from build123d import *

# Parameters (mm, degrees)
IZIM1_W                     = 15
IZIM1_H                     = 153
Y_KSEKLIK_EKSTR_ZYON1_DEPTH = 100
IZIM2_R                     = 5
KES_EKSTR_ZYON2_DEPTH       = 16
IZIM3_R                     = 16
KES_EKSTR_ZYON3_DEPTH       = 16


with BuildPart() as part:
    # Çizim1 → Yükseklik-Ekstrüzyon1 (new body)
    with BuildSketch(Plane.XY):
        Rectangle(IZIM1_W, IZIM1_H)
    extrude(amount=Y_KSEKLIK_EKSTR_ZYON1_DEPTH)

    # Çizim2 → Kes-Ekstrüzyon2 (cut, through all)
    with BuildSketch(Plane(origin=(7.5, 0, 0), x_dir=(0, 0, -1), z_dir=(1, 0, 0))):
        with Locations((-75, -69)):
            Circle(IZIM2_R)
        with Locations((-25, -69)):
            Circle(IZIM2_R)
    extrude(amount=-KES_EKSTR_ZYON2_DEPTH, mode=Mode.SUBTRACT)

    # Çizim3 → Kes-Ekstrüzyon3 (cut, through all)
    with BuildSketch(Plane(origin=(7.5, 0, 0), x_dir=(0, 0, -1), z_dir=(1, 0, 0))):
        with Locations((-50, -21.5)):
            Circle(IZIM3_R)
        with BuildLine():
            Line((-58.38409441, 35.653702621), (-41.38409441, 35.653702621))
            ThreePointArc((-41.38409441, 35.653702621), (-37.848560504, 37.118168715), (-36.38409441, 40.653702621))
            Line((-36.38409441, 40.653702621), (-36.38409441, 57.653702621))
            ThreePointArc((-36.38409441, 57.653702621), (-37.848560504, 61.189236527), (-41.38409441, 62.653702621))
            Line((-41.38409441, 62.653702621), (-58.38409441, 62.653702621))
            ThreePointArc((-58.38409441, 62.653702621), (-61.919628316, 61.189236527), (-63.38409441, 57.653702621))
            Line((-63.38409441, 57.653702621), (-63.38409441, 40.653702621))
            ThreePointArc((-63.38409441, 40.653702621), (-61.919628316, 37.118168715), (-58.38409441, 35.653702621))
        make_face()
    extrude(amount=-KES_EKSTR_ZYON3_DEPTH, mode=Mode.SUBTRACT)


solid = part.part
Could you check a few things on this model? Use its own coordinates, in mm. A direction names the side the tool comes from. Give positions to 0.01 mm unless a question says otherwise; leave off trailing zeros. Loops run counter-clockwise (first coordinate to the right, second up) from the corner with the lowest first, then second, coordinate; pieces in that order, holes last. Notation, with made-up numbers: M -34.75,88.25 L 18.25,88.25 A22 cw 18.25,108.25 Z; hole C 53.5,19.25 d1. An arc over 180 degrees is marked long. Answer as a JSON object with one key per item and string values.
Q1. Suppose I cut it at A-A, the plane z = 50. List the corners of the cut face in (x, y) for me.
Values found:
{"outline": "M -7.5,-76.5 L 7.5,-76.5 L 7.5,-37.5 L -7.5,-37.5 Z; M -7.5,-5.5 L 7.5,-5.5 L 7.5,35.65 L -7.5,35.65 Z; M -7.5,62.65 L 7.5,62.65 L 7.5,76.5 L -7.5,76.5 Z"}
Q2. For faces 4 (the flat face through (-7.5, -1, 49)), 5 (the cylindrical face through (0.11, 37.08, 37.89)), which set-ups out of +Z, -Z, +X, -X, +Y, -Y let a thin tool reach every point of the face, with its end or its side?
Values found:
{"face 4": "+Z, -Z, -X, +Y, -Y", "face 5": "+X, -X"}
Q3. For P1, Ø4, axis at x = -5.5, y = 33, coming from the -Z side, with a flat end and sliding along its axis, tell me the tip position at first contact or that it passes through.
Values found:
{"P1": "stops at z = 0"}
Q4. If we mould it in two halves opening along Z, with no side actions, what happens to faces 1 (the flat face through (0, 49, 36.384)), 2 (the flat face through (0, 1, 0)), 3 (the flat face through (0, 76.5, 49))? For each: pulls with the +Z half, pulls with the -Z half, needs draft (parallel to the pull), parting line crosses it, or undercut.
Values found:
{"face 1": "undercut", "face 2": "pulls with the -Z half", "face 3": "needs draft"}
Q5. Suppose I cut it at D-D, the plane x = -5.25. List the corners of the cut face in (y, z) for me.
Values found:
{"outline": "M -76.5,0 L 76.5,0 L 76.5,100 L -76.5,100 Z; hole C -69,25 d10; hole C -69,75 d10; hole C -21.5,50 d32; hole M 35.65,41.38 A5 ccw 40.65,36.38 L 57.65,36.38 A5 ccw 62.65,41.38 L 62.65,58.38 A5 ccw 57.65,63.38 L 40.65,63.38 A5 ccw 35.65,58.38 Z"}
Q6. If I drill on probe 1 along Y at (x, z) = (3.25, 50); probe 2 along Y at (x, z) = (-1, 41.5); probe 3 along Y at (x, z) = (3.25, 25), over which ranges is the centre line in solid material (lowest first)? Write a range as [from, to].
Values found:
{"probe 1": "y = [-76.5, -37.5], [-5.5, 35.65], [62.65, 76.5]", "probe 2": "y = [-76.5, -35.06], [-7.94, 35.65], [62.65, 76.5]", "probe 3": "y = [-76.5, -74], [-64, 76.5]"}
Q7. Suppose I cut it at C-C, the plane z = 28. List the corners of the cut face in (x, y) for me.
Values found:
{"outline": "M -7.5,-76.5 L 7.5,-76.5 L 7.5,-73 L -7.5,-73 Z; M -7.5,-65 L 7.5,-65 L 7.5,76.5 L -7.5,76.5 Z"}
Q8. Suppose I cut it at B-B, the plane y = -69. List the corners of the cut face in (x, z) for me, plus the area to 3 significant figures.
Values found:
{"outline": "M -7.5,0 L 7.5,0 L 7.5,20 L -7.5,20 Z; M -7.5,30 L 7.5,30 L 7.5,70 L -7.5,70 Z; M -7.5,80 L 7.5,80 L 7.5,100 L -7.5,100 Z", "area": "1,200 mm²"}
